from build123d import *

# Parameters (mm, degrees)
F1_DEPTH = 5
F2_DEPTH = 5
F3_DEPTH = 132
F4_DEPTH = 132
F5_DEPTH = 259


with BuildPart() as f1:
    # F0 (on Top) → F1 (new body)
    with BuildSketch(Plane.XY):
        with BuildLine():
            ThreePointArc((20, -82.6135582093), (66.8019460794, -52.5594901041), (85, 0))
            ThreePointArc((85, 0), (66.8019460794, 52.5594901041), (20, 82.6135582093))
            ThreePointArc((20, 82.6135582093), (10.0709372009, 84.4012809375), (0, 85))
            ThreePointArc((0, 85), (-85, 0), (0, -85))
            ThreePointArc((0, -85), (10.0709372009, -84.4012809375), (20, -82.6135582093))
        make_face()
    extrude(amount=F1_DEPTH)

    # F0 (on Top) → F2 (join)
    with BuildSketch(Plane.XY):
        with BuildLine():
            ThreePointArc((0, 85), (10.0709372009, 84.4012809375), (20, 82.6135582093))
            Line((20, 82.6135582093), (20, 85))
            Line((20, 85), (0, 85))
        make_face()
        with BuildLine():
            Line((20, -85), (20, -82.6135582093))
            ThreePointArc((20, -82.6135582093), (10.0709372009, -84.4012809375), (0, -85))
            Line((0, -85), (20, -85))
        make_face()
    extrude(amount=F2_DEPTH)

    # F0 (on Top) → F3 (join)
    with BuildSketch(Plane.XY):
        with BuildLine():
            ThreePointArc((170, -85), (109.8959235991, -60.1040764009), (85, 0))
            ThreePointArc((85, 0), (66.8019460794, -52.5594901041), (20, -82.6135582093))
            Line((20, -82.6135582093), (20, -85))
            Line((20, -85), (170, -85))
        make_face()
        with BuildLine():
            ThreePointArc((20, 82.6135582093), (66.8019460794, 52.5594901041), (85, 0))
            ThreePointArc((85, 0), (109.8959235991, 60.1040764009), (170, 85))
            Line((170, 85), (20, 85))
            Line((20, 85), (20, 82.6135582093))
        make_face()
        with BuildLine():
            ThreePointArc((170, 85), (109.8959235991, 60.1040764009), (85, 0))
            ThreePointArc((85, 0), (109.8959235991, -60.1040764009), (170, -85))
            ThreePointArc((170, -85), (180.0709372009, -84.4012809375), (190, -82.6135582093))
            ThreePointArc((190, -82.6135582093), (236.8019460794, -52.5594901041), (255, 0))
            ThreePointArc((255, 0), (236.8019460794, 52.5594901041), (190, 82.6135582093))
            ThreePointArc((190, 82.6135582093), (180.0709372009, 84.4012809375), (170, 85))
        make_face()
    extrude(amount=F3_DEPTH)

    # F0 (on Top) → F4 (join)
    with BuildSketch(Plane.XY):
        with BuildLine():
            Line((190, 85), (170, 85))
            ThreePointArc((170, 85), (180.0709372009, 84.4012809375), (190, 82.6135582093))
            Line((190, 82.6135582093), (190, 85))
        make_face()
        with BuildLine():
            ThreePointArc((190, -82.6135582093), (180.0709372009, -84.4012809375), (170, -85))
            Line((170, -85), (190, -85))
            Line((190, -85), (190, -82.6135582093))
        make_face()
    extrude(amount=F4_DEPTH)

    # F0 (on Top) → F5 (join)
    with BuildSketch(Plane.XY):
        with BuildLine():
            Line((248.512, 85), (190, 85))
            Line((190, 85), (190, 82.6135582093))
            ThreePointArc((190, 82.6135582093), (236.8019460794, 52.5594901041), (255, 0))
            ThreePointArc((255, 0), (236.8019460794, -52.5594901041), (190, -82.6135582093))
            Line((190, -82.6135582093), (190, -85))
            Line((190, -85), (248.512, -85))
            Line((248.512, -85), (278.512, -85))
            Line((278.512, -85), (278.512, 85))
            Line((278.512, 85), (248.512, 85))
        make_face()
    extrude(amount=F5_DEPTH)


solid = f1.part
CAD build for the part. Positions are in the model's coordinates, mm. A direction names the side the tool comes from. Coordinates: 2 decimals unless noted, no trailing zeros. Order: outer loops, then holes, each group sorted by start corner. A loop starts at its lowest first (then second) coordinate and runs counter-clockwise, first axis right, second up. Notation, with made-up numbers: (76, 37) -> (98, 37) arc R20 ccw to (98, 43) -> close; hole circle Ø8 at (76.25, -13.5). An arc over 180 degrees is marked (long way). Answer in a Markdown table with one row per item.
1) Band-saw the part on A-A (y = 0). List the corners of the cut face in (x, z).
Check values:
| item | result |
|---|---|
| outline | (-85, 0) -> (278.51, 0) -> (278.51, 259) -> (255, 259) -> (255, 132) -> (85, 132) -> (85, 5) -> (-85, 5) -> close |
2) Band-saw the part on D-D (z = 184). List the corners of the cut face in (x, y).
Check values:
| item | result |
|---|---|
| outline | (190, -85) -> (278.51, -85) -> (278.51, 85) -> (190, 85) -> (190, 82.61) arc R85 cw to (190, -82.61) -> close |
3) Drill centre lines: line 1 (Z direction, x = 176, y = -74); line 2 (Z direction, x = -29, y = 62.5); line 3 (X direction, y = -1, z = 147). Where is each one in solid material? Low to high.
Check values:
| item | result |
|---|---|
| line 1 | 0 to 132 |
| line 2 | 0 to 5 |
| line 3 | 254.99 to 278.51 |
4) Flat gauge pins, fed straight in: P1, Ø6, axis at x = 74, y = -9, coming from the +Z side; P2, Ø2.5, axis at y = -84, z = 170.5, coming from the -X side; P3, Ø1.9, axis at y = -83.5, z = 39.5, coming from the -X side. Where does each tip first touch, or does it go through?
Check values:
| item | result |
|---|---|
| P1 | z = 5 |
| P2 | x = 190 |
| P3 | x = 20 |
5) Which spindle directions (+Z, -Z, +X, -X, +Y, -Y) get a long thin tool onto all of the face, cutting with end or side? Do faces 4 (the face through (254.985, 1.587, 194.611)), 5 (the face through (172, 85, 99)). Say none if no direction does.
Check values:
| item | result |
|---|---|
| face 4 | +Z, -X |
| face 5 | +Z, -Z, +X, -X, +Y |
6) Band-saw the part on B-B (x = 50). List the corners of the cut face in (y, z).
Check values:
| item | result |
|---|---|
| outline | (-85, 0) -> (85, 0) -> (85, 132) -> (68.74, 132) -> (68.74, 5) -> (-68.74, 5) -> (-68.74, 132) -> (-85, 132) -> close |
7) Band-saw the part on C-C (z = 62). List the corners of the cut face in (x, y), and give its area (3 significant figures).
Check values:
| item | result |
|---|---|
| outline | (20, -85) -> (278.51, -85) -> (278.51, 85) -> (20, 85) -> (20, 82.61) arc R85 cw to (20, -82.61) -> close |
| area | 36,000 mm2 |
8) Mould opens along Y. For faces 1 (the face through (168, -85, 99)), 2 (the face through (94, 1, 0)), 3 (the face through (162, 1, 132)) say: pulls with the +Y half, pulls with the -Y half, needs draft (parallel to the pull), parting line crosses it, or undercut.
Check values:
| item | result |
|---|---|
| face 1 | pulls with the -Y half |
| face 2 | needs draft |
| face 3 | undercut |
